Read the model definition and answer for the solid it produces. Units are mm, in the model's axes. Coordinates: 2 decimals unless noted, no trailing zeros. Write each loop counter-clockwise with the first axis right and the second up, starting at its lowest first coordinate (ties: lowest second). Pieces come first, ordered by that corner, then holes.
(1) Given pin 1 (1.5 mm diameter, centred on x = -2, z = -9, fed in from -Y); pin 2 (1.8 mm diameter, centred on x = -1.5, z = -21.5, fed in from +Y); pin 3 (3 mm diameter, centred on x = -1, z = -22.5, fed in from -Y), each flat-ended and moving along its own axis, determine where each tip first touches the part or whether it passes through.
(2) Find the intervals of material crossed by probe 1 along Z at (x, y) = (0, 0.55); probe 2 along X at (y, z) = (0, -22); probe 3 along Y at (x, z) = (-0.25, -19), in increasing order.
(3) Section A-A on z = -7 is taken. Write down the section's boundary in (x, y), then the cut area to 3 significant figures.
(4) Section B-B on z = -17 is taken. Write down the section's boundary in (x, y).
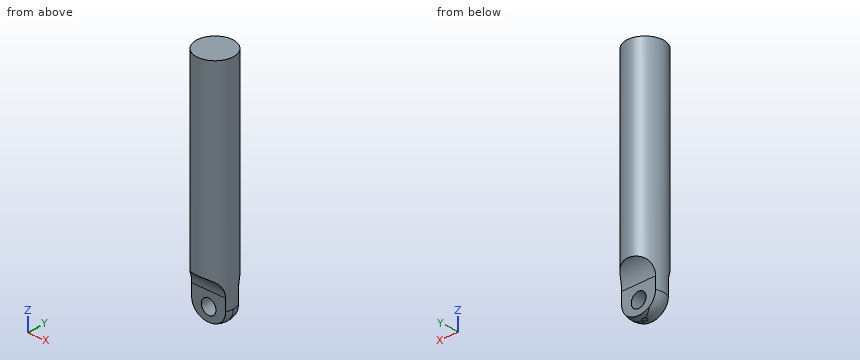
from build123d import *

# Parameters (mm, degrees)
SKETCH1_R               = 4
BOSS_EXTRUDE1_DEPTH     = 25
CUT_EXTRUDE1_DEPTH      = 26.632011236
CUT_EXTRUDE1_DEPTH_BACK = 26.632011236
SKETCH2_W               = 10
SKETCH2_H               = 2.5
FILLET1_R               = 4
M3_CLEARANCE_HOLE1_D    = 3.2
FILLET2_R               = 3.5


with BuildPart() as part:
    # Sketch1 → Boss-Extrude1 (new, symmetric)
    with BuildSketch(Plane.XY):
        Circle(SKETCH1_R)
    extrude(amount=BOSS_EXTRUDE1_DEPTH, both=True)

    # Sketch2 → Cut-Extrude1 (cut, two sides: drawn at the far end of the back side and taken through both)
    with BuildSketch(Plane(origin=(0, 0, 0), x_dir=(0, 0, -1), z_dir=(1, 0, 0)).offset(-CUT_EXTRUDE1_DEPTH_BACK)):
        with Locations((20, -2.75)):
            Rectangle(SKETCH2_W, SKETCH2_H)
        with Locations((20, 2.75)):
            Rectangle(SKETCH2_W, SKETCH2_H)
    extrude(amount=CUT_EXTRUDE1_DEPTH + CUT_EXTRUDE1_DEPTH_BACK, mode=Mode.SUBTRACT)

    # Fillet1
    # the kernel refuses this fillet: 4 mm, written as the material it adds along each edge
    with BuildSketch(Plane(origin=(13.708099244, -1.5, -15), x_dir=(0, -1, 0), z_dir=(-1, 0, 0))) as fillet1_piece_1_section:
        with BuildLine():
            CenterArc((FILLET1_R, -FILLET1_R), FILLET1_R, 90, 90)
            Line((0, -FILLET1_R), (0, 0))
            Line((0, 0), (FILLET1_R, 0))
        make_face()
    fillet1_piece_1 = extrude(amount=27.416198487, mode=Mode.PRIVATE)
    fillet1_piece_1 = fillet1_piece_1 & Plane(origin=(0, 0, -16.053491098), x_dir=(1, 0, 0), z_dir=(0, 0, 1)) * Cylinder(4, 71, mode=Mode.PRIVATE)
    add(fillet1_piece_1)
    with BuildSketch(Plane(origin=(-13.708099244, 1.5, -15), x_dir=(0, 1, 0), z_dir=(1, 0, 0))) as fillet1_piece_2_section:
        with BuildLine():
            CenterArc((FILLET1_R, -FILLET1_R), FILLET1_R, 90, 90)
            Line((0, -FILLET1_R), (0, 0))
            Line((0, 0), (FILLET1_R, 0))
        make_face()
    fillet1_piece_2 = extrude(amount=27.416198487, mode=Mode.PRIVATE)
    fillet1_piece_2 = fillet1_piece_2 & Plane(origin=(0, 0, -16.053491097), x_dir=(1, 0, 0), z_dir=(0, 0, 1)) * Cylinder(4, 71, mode=Mode.PRIVATE)
    add(fillet1_piece_2)

    # M3 Clearance Hole1 (through all)
    with Locations(Plane(origin=(0, 1.5, 0), x_dir=(1, 0, 0), z_dir=(0, 1, 0))):
        with Locations((0, 22)):
            Hole(M3_CLEARANCE_HOLE1_D / 2)

    # Fillet2
    # the kernel refuses this fillet: 3.5 mm, written as the material it takes off along each edge
    with BuildSketch(Plane(origin=(0, 0, -25), x_dir=(1, 0, 0), z_dir=(0, -1, 0))) as fillet2_piece_1:
        with BuildLine():
            CenterArc((4 - FILLET2_R, FILLET2_R), FILLET2_R, 270, 90)
            Line((4 - FILLET2_R, 0), (4, 0))
            Line((4, 0), (4, FILLET2_R))
        make_face()
    revolve(axis=Axis((0, 0, -25), (0, 0, 1)), revolution_arc=147.36184482, mode=Mode.SUBTRACT)
    with BuildSketch(Plane(origin=(0, 0, -25), x_dir=(0.842178541761355, 0.5391987609376692, 0), z_dir=(0.5391987609376692, -0.842178541761355, 0))) as fillet2_piece_2:
        with BuildLine():
            CenterArc((4 - FILLET2_R, FILLET2_R), FILLET2_R, 270, 90)
            Line((4 - FILLET2_R, 0), (4, 0))
            Line((4, 0), (4, FILLET2_R))
        make_face()
    revolve(axis=Axis((0, 0, -25), (0, 0, 1)), revolution_arc=294.74177665, mode=Mode.SUBTRACT)
    with BuildSketch(Plane(origin=(0, 0, -25), x_dir=(-0.8420934247140166, -0.5393316827828853, 0), z_dir=(-0.5393316827828853, 0.8420934247140166, 0))) as fillet2_piece_3:
        with BuildLine():
            CenterArc((4 - FILLET2_R, FILLET2_R), FILLET2_R, 270, 90)
            Line((4 - FILLET2_R, 0), (4, 0))
            Line((4, 0), (4, FILLET2_R))
        make_face()
    revolve(axis=Axis((0, 0, -25), (0, 0, 1)), revolution_arc=147.36184482, mode=Mode.SUBTRACT)


solid = part.part
Response:
1. pin 1: stops at y = -3.8
1. pin 2: stops at y = 1.5
1. pin 3: stops at y = -1.5
2. probe 1: z = -25 to -23.6, -20.4 to 25
2. probe 2: x = -3.96 to -1.6, 1.6 to 3.96
2. probe 3: y = -1.5 to 1.5
3. outline: circle Ø8 at (0, 0)
3. area: 50.3 mm2
4. outline: (-3.44, -2.04) - (3.44, -2.04) arc R4 ccw to (3.44, 2.04) - (-3.44, 2.04) arc R4 ccw to start
